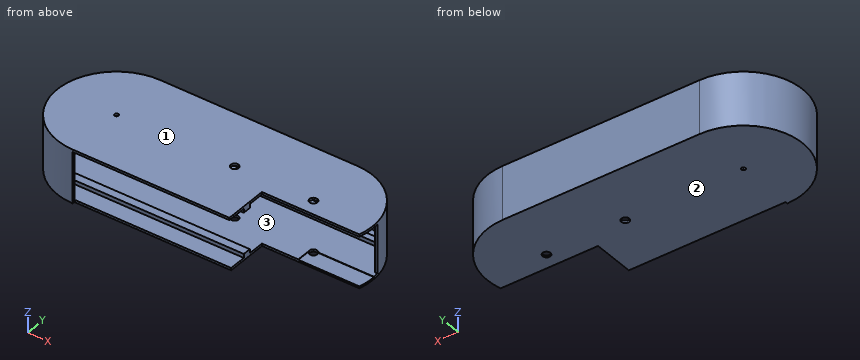
from build123d import *

# Parameters (mm, degrees)
EXTRUDE_1_DEPTH          = 68
CUT_EXTRUDE_2_DEPTH      = 62
SKETCH_3_W               = 250
SKETCH_3_H               = 65
CUT_EXTRUDE_3_DEPTH      = 3
CUT_EXTRUDE_5_DEPTH      = 340.816126751
CUT_EXTRUDE_5_DEPTH_BACK = 340.816126751
CUT_EXTRUDE_6_DEPTH      = 340.816126751
CUT_EXTRUDE_6_DEPTH_BACK = 340.816126751
SKETCH_5_R               = 5
SKETCH_6_W               = 62.5
SKETCH_6_H               = 77.5
CUT_EXTRUDE_7_DEPTH      = 80
CUT_EXTRUDE_8_DEPTH      = 340.816126751
CUT_EXTRUDE_8_DEPTH_BACK = 340.816126751
SKETCH_7_W               = 123.617687057
SKETCH_7_H               = 55.714084123
SKETCH_8_R               = 5
EXTRUDE_2_DEPTH          = 6
EXTRUDE_START            = 6
EXTRUDE_3_DEPTH          = 6
EXTRUDE_4_DEPTH          = 5
PATTERN_LINEAR_1_COUNT   = 2
PATTERN_LINEAR_1_PITCH   = 57
SKETCH_12_W              = 62
SKETCH_12_H              = 9.024181297
CUT_EXTRUDE_9_DEPTH      = 10


with BuildPart() as part:
    # 草图1 → 凸台-拉伸1 (new body)
    with BuildSketch(Plane.XY):
        with BuildLine():
            Line((0, 75), (250, 75))
            ThreePointArc((250, 75), (325, 0), (250, -75))
            Line((250, -75), (0, -75))
            ThreePointArc((0, -75), (-75, 0), (0, 75))
        make_face()
    extrude(amount=EXTRUDE_1_DEPTH)

    # 草图2 → 切除-拉伸2 (cut)
    with BuildSketch(Plane.XY.offset(65)):
        with BuildLine():
            Line((0, 72), (250, 72))
            ThreePointArc((250, 72), (322, 0), (250, -72))
            Line((250, -72), (0, -72))
            ThreePointArc((0, -72), (-72, 0), (0, 72))
        make_face()
    extrude(amount=-CUT_EXTRUDE_2_DEPTH, mode=Mode.SUBTRACT)

    # 草图3 → 切除-拉伸3 (cut)
    with BuildSketch(Plane(origin=(0, -75, 0), x_dir=(-1, 0, 0), z_dir=(0, -1, 0))):
        with Locations((-125, -32.5)):
            Rectangle(SKETCH_3_W, SKETCH_3_H)
    extrude(amount=-CUT_EXTRUDE_3_DEPTH, mode=Mode.SUBTRACT)

    # 草图4 → 切除-拉伸5 (cut, two sides: drawn at the far end of the back side and taken through both)
    with BuildSketch(Plane.XY.offset(65).offset(-CUT_EXTRUDE_5_DEPTH_BACK)):
        with BuildLine():
            ThreePointArc((2.5, 0), (1.767766953, 1.767766953), (0, 2.5))
            Line((0, 2.5), (0, -2.5))
            ThreePointArc((0, -2.5), (1.767766953, -1.767766953), (2.5, 0))
        make_face()
        with BuildLine():
            Line((0, -2.5), (0, 2.5))
            ThreePointArc((0, 2.5), (-2.5, 0), (0, -2.5))
        make_face()
    extrude(amount=CUT_EXTRUDE_5_DEPTH + CUT_EXTRUDE_5_DEPTH_BACK, mode=Mode.SUBTRACT)

    # 草图5 → 切除-拉伸6 (cut, two sides: drawn at the far end of the back side and taken through both)
    with BuildSketch(Plane.XY.offset(65).offset(-CUT_EXTRUDE_6_DEPTH_BACK)):
        with Locations((250, 0)):
            Circle(SKETCH_5_R)
        with Locations((150, 0)):
            Circle(SKETCH_5_R)
    extrude(amount=CUT_EXTRUDE_6_DEPTH + CUT_EXTRUDE_6_DEPTH_BACK, mode=Mode.SUBTRACT)

    # 草图6 → 切除-拉伸7 (cut)
    with BuildSketch(Plane(origin=(325, 0, 0), x_dir=(0, 0, -1), z_dir=(1, 0, 0))):
        with Locations((-33.75, -36.25)):
            Rectangle(SKETCH_6_W, SKETCH_6_H)
    extrude(amount=-CUT_EXTRUDE_7_DEPTH, mode=Mode.SUBTRACT)

    # 草图7 → 切除-拉伸8 (cut, two sides: drawn at the far end of the back side and taken through both)
    with BuildSketch(Plane.XY.offset(65).offset(-CUT_EXTRUDE_8_DEPTH_BACK)):
        with Locations((260.669107939, -47.142957939)):
            Rectangle(SKETCH_7_W, SKETCH_7_H)
    extrude(amount=CUT_EXTRUDE_8_DEPTH + CUT_EXTRUDE_8_DEPTH_BACK, mode=Mode.SUBTRACT)

    # 草图8 → 凸台-拉伸2 (add)
    with BuildSketch(Plane(origin=(0, 0, 65), x_dir=(-1, 0, 0), z_dir=(0, 0, -1))):
        with Locations(Location((-32.64, 0, 0), (0, 0, 180))):
            Circle(SKETCH_8_R)
    extrude(amount=EXTRUDE_2_DEPTH)

    # 草图9 → 凸台-拉伸3 (add)
    with BuildSketch(Plane.XY.offset(3).offset(EXTRUDE_START)):
        with BuildLine():
            ThreePointArc((37.64, 0), (32.64, 5), (27.64, 0))
            Line((27.64, 0), (37.64, 0))
        make_face()
        with BuildLine():
            Line((37.64, 0), (27.64, 0))
            ThreePointArc((27.64, 0), (32.64, -5), (37.64, 0))
        make_face()
    extrude(amount=-EXTRUDE_3_DEPTH)

    # 草图10 → 凸台-拉伸4 (add)
    with BuildSketch(Plane.XY.offset(3)):
        Polygon((-52.288307715, 53.767396034), (302.288307715, 53.767396034), (309.461936105, 45.708622323), (-58.724061421, 46.652809243), align=None)
        Polygon((-63.45501943, -39.980751734), (198.86026441, -39.980751734), (198.86026441, -50.331270565), (-55.603625811, -50.331270565), align=None)
    extrude_4 = extrude(amount=EXTRUDE_4_DEPTH)

    # 阵列(线性)1: 凸台-拉伸4 ×2
    with Locations(*[(0, 0, i * PATTERN_LINEAR_1_PITCH) for i in range(1, PATTERN_LINEAR_1_COUNT)]):
        add(extrude_4)

    # 草图12 → 切除-拉伸9 (cut)
    with BuildSketch(Plane(origin=(325, 0, 0), x_dir=(0, 0, -1), z_dir=(1, 0, 0))):
        with Locations((-34, 4.512090649)):
            Rectangle(SKETCH_12_W, SKETCH_12_H)
    extrude(amount=-CUT_EXTRUDE_9_DEPTH, mode=Mode.SUBTRACT)


solid = part.part
Source: CAD feature listing. Evaluate the final solid. Frame: model axes, mm. Face numbers are marked on the shaded views. Coordinates: 2 decimals unless noted, no trailing zeros. Order: outer loops, then holes, each group sorted by start corner. A loop starts at its lowest first (then second) coordinate and runs counter-clockwise, first axis right, second up. Notation, with made-up numbers: M 68.5,-28.5 L 72.5,-28.5 A15 cw 72.5,-5.5 Z; hole C 33.5,6 d5. An arc over 180 degrees is marked long. Write each question's results on one line, items separated by ' | '. Start each with the question number.
1. Pin query (flat end, axial travel): pin 1 (1.5 mm diameter, centred on x = 62, y = -40.5, fed in from -Z); pin 2 (9 mm diameter, centred on y = -39.5, z = 63.5, fed in from +X); pin 3 (1.5 mm diameter, centred on x = 322.5, z = 26, fed in from -Y); pin 4 (4 mm diameter, centred on y = 21.5, z = 12.5, fed in from -X). Return the tip coordinate at first contact, or that it passes through.
2. Material intervals for L1, parallel to X at y = 0, z = 67.15; L2, parallel to Z at x = 52.5, y = 22; L3, parallel to Y at x = 250, z = 66.6, sorted ascending.
3. Section A-A, the plane z = 26. Return the cut outline in (x, y).
4. Draft query along Z for the marked faces 1, 2 and 3. Return one class per face: +Z half, -Z half, draft (parallel to the pull), parting line (faces both ways), or undercut.
Solution:
1) pin 1: z = 0 | pin 2: x = 198.86 | pin 3: y = 9.02 | pin 4: x = -72.42
2) L1: -75 to -2.5, 2.5 to 145, 155 to 245, 255 to 325 | L2: 0 to 3, 65 to 68 | L3: -19.29 to -5, 5 to 75
3) outline: M 0,-75 L 0,-72 A72 cw 0,72 L 250,72 A72 cw 321.43,9.02 L 324.46,9.02 A75 ccw 250,75 L 0,75 A75 ccw Z
4) face 1: +Z half | face 2: -Z half | face 3: undercut
